For this review, use the dimensioned drawing (mm, ordinates from the lowest corner) and the shaded views. A direction names the side the tool comes from. Coordinates: 2 decimals unless noted, no trailing zeros. Order: outer loops, then holes, each group sorted by start corner. A loop starts at its lowest first (then second) coordinate and runs counter-clockwise, first axis right, second up. Notation, with made-up numbers: M 32.5,19 L 82.5,19 A25 ccw 82.5,34 Z; hole C 77,74.25 d4. An arc over 180 degrees is marked long. One line per item, written item: value.
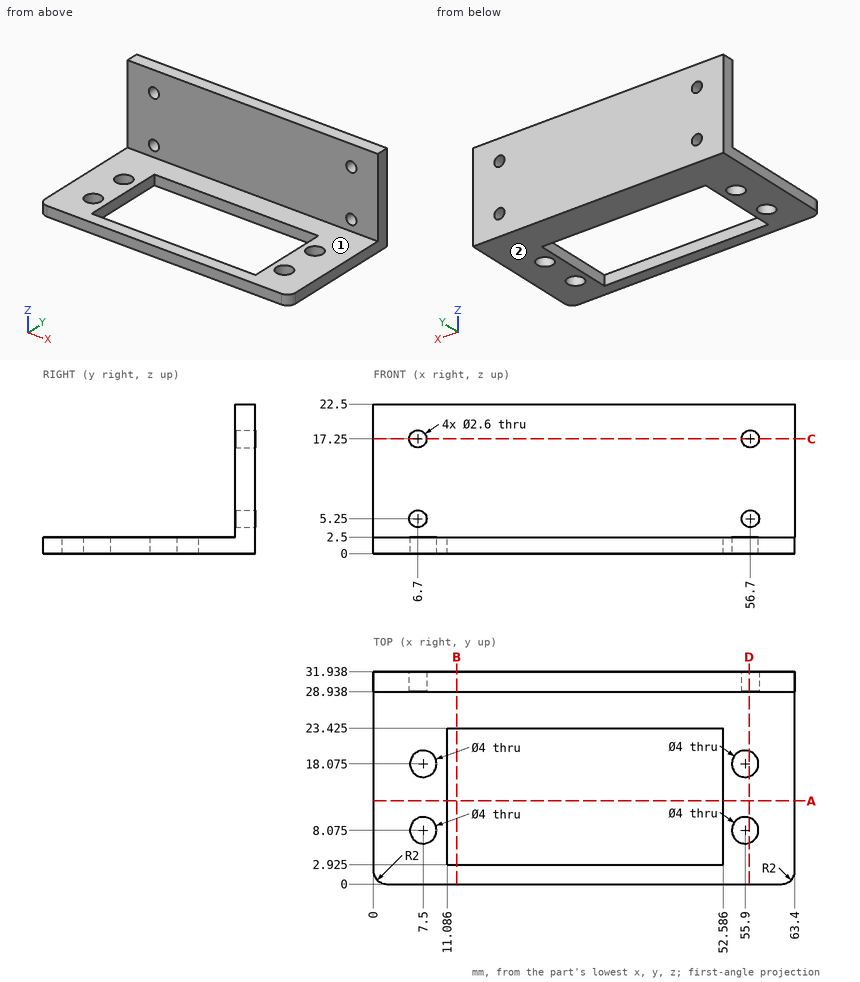
(1) We need section A-A, the plane y = 12.5. State the section outline as (x, z) points (1 decimal).
Geometry results:
outline: M 0,0 L 11.1,0 L 11.1,2.5 L 0,2.5 Z; M 52.6,0 L 63.4,0 L 63.4,2.5 L 52.6,2.5 Z
(2) Tool access review of the marked faces 1 and 2: name each direction out of +Z, -Z, +X, -X, +Y, -Y from which nothing blocks a thin tool from reaching the whole face with its end or side.
Geometry results:
face 1: +Z, +X, -X, -Y
face 2: -Z, +X, -X, +Y, -Y
(3) We need section C-C, the plane z = 17.25. State the section outline as (x, y) points.
Geometry results:
outline: M 0,28.94 L 5.4,28.94 L 5.4,31.94 L 0,31.94 Z; M 8,28.94 L 55.4,28.94 L 55.4,31.94 L 8,31.94 Z; M 58,28.94 L 63.4,28.94 L 63.4,31.94 L 58,31.94 Z
(4) We need section B-B, the plane x = 12.5. State the section outline as (y, z) points (1 decimal).
Geometry results:
outline: M 0,0 L 2.9,0 L 2.9,2.5 L 0,2.5 Z; M 23.4,0 L 31.9,0 L 31.9,22.5 L 28.9,22.5 L 28.9,2.5 L 23.4,2.5 Z
(5) Insertion check: pin 1 Ø10 at (x, z) = (32.5, 17.5) entering from -Y; pin 2 Ø5 at (x, y) = (55.9, 8.08) entering from +Z. Each pin has a flat end and moves straight along its axis. Give the tip position at first contact, or say it passes through.
Geometry results:
pin 1: stops at y = 28.94
pin 2: stops at z = 2.5
(6) We need section D-D, the plane x = 56.5. State the section outline as (y, z) points (1 decimal).
Geometry results:
outline: M 0,0 L 6.2,0 L 6.2,2.5 L 0,2.5 Z; M 10,0 L 16.2,0 L 16.2,2.5 L 10,2.5 Z; M 20,0 L 31.9,0 L 31.9,4 L 28.9,4 L 28.9,2.5 L 20,2.5 Z; M 28.9,6.5 L 31.9,6.5 L 31.9,16 L 28.9,16 Z; M 28.9,18.5 L 31.9,18.5 L 31.9,22.5 L 28.9,22.5 Z
(7) For L1, parallel to X at y = 30.3, z = 5.25; L2, parallel to X at y = 7, z = 1.75 (1 decimal); L3, parallel to Z at x = 3, y = 25, list the stretches that pass through material, from the lowest coordinate up.
Geometry results:
L1: x = 0 to 5.4, 8 to 55.4, 58 to 63.4
L2: x = 0 to 5.8, 9.2 to 11.1, 52.6 to 54.2, 57.6 to 63.4
L3: z = 0 to 2.5
